from build123d import *

# Parameters (mm, degrees)
EXTRUDE_1_DEPTH = 3


with BuildPart() as part:
    # 草图1 → 凸台-拉伸1 (new body)
    with BuildSketch(Plane.XY):
        with BuildLine():
            Line((100.55, -11), (100.55, 11))
            Line((100.55, 11), (93.45, 11))
            ThreePointArc((93.45, 11), (92.4, 12.05), (93.45, 13.1))
            Line((93.45, 13.1), (93.45, 16))
            Line((93.45, 16), (49.05, 16))
            Line((49.05, 16), (49.05, 15.2))
            ThreePointArc((49.05, 15.2), (49.79246212, 14.89246212), (50.1, 14.15))
            ThreePointArc((50.1, 14.15), (49.79246212, 13.40753788), (49.05, 13.1))
            Line((49.05, 13.1), (45.95, 13.1))
            ThreePointArc((45.95, 13.1), (44.9, 14.15), (45.95, 15.2))
            Line((45.95, 15.2), (45.95, 16))
            Line((45.95, 16), (1.55, 16))
            Line((1.55, 16), (1.55, 13.1))
            ThreePointArc((1.55, 13.1), (2.29246212, 12.79246212), (2.6, 12.05))
            ThreePointArc((2.6, 12.05), (2.29246212, 11.30753788), (1.55, 11))
            Line((1.55, 11), (-5.55, 11))
            Line((-5.55, 11), (-5.55, -11))
            Line((-5.55, -11), (1.55, -11))
            ThreePointArc((1.55, -11), (2.29246212, -11.30753788), (2.6, -12.05))
            ThreePointArc((2.6, -12.05), (2.29246212, -12.79246212), (1.55, -13.1))
            Line((1.55, -13.1), (1.55, -16))
            Line((1.55, -16), (45.95, -16))
            Line((45.95, -16), (45.95, -15.2))
            ThreePointArc((45.95, -15.2), (44.9, -14.15), (45.95, -13.1))
            Line((45.95, -13.1), (49.05, -13.1))
            ThreePointArc((49.05, -13.1), (49.79246212, -13.40753788), (50.1, -14.15))
            ThreePointArc((50.1, -14.15), (49.79246212, -14.89246212), (49.05, -15.2))
            Line((49.05, -15.2), (49.05, -16))
            Line((49.05, -16), (93.45, -16))
            Line((93.45, -16), (93.45, -13.1))
            ThreePointArc((93.45, -13.1), (92.4, -12.05), (93.45, -11))
            Line((93.45, -11), (100.55, -11))
        make_face()
        with BuildLine():
            ThreePointArc((2.6, -4.05), (2.29246212, -4.79246212), (1.55, -5.1))
            Line((1.55, -5.1), (-1.55, -5.1))
            ThreePointArc((-1.55, -5.1), (-2.6, -4.05), (-1.55, -3))
            Line((-1.55, -3), (-1.55, 3))
            ThreePointArc((-1.55, 3), (-2.6, 4.05), (-1.55, 5.1))
            Line((-1.55, 5.1), (1.55, 5.1))
            ThreePointArc((1.55, 5.1), (2.29246212, 4.79246212), (2.6, 4.05))
            ThreePointArc((2.6, 4.05), (2.29246212, 3.30753788), (1.55, 3))
            Line((1.55, 3), (1.55, -3))
            ThreePointArc((1.55, -3), (2.29246212, -3.30753788), (2.6, -4.05))
        make_face(mode=Mode.SUBTRACT)
        Polygon((39.300498915, -12.5), (8.199501085, -12.5), (23.75, -1.819712284), align=None, mode=Mode.SUBTRACT)
        Polygon((55.699501085, -12.5), (71.25, -1.819712284), (86.800498915, -12.5), align=None, mode=Mode.SUBTRACT)
        with BuildLine():
            ThreePointArc((97.6, -4.05), (97.29246212, -4.79246212), (96.55, -5.1))
            Line((96.55, -5.1), (93.45, -5.1))
            ThreePointArc((93.45, -5.1), (92.4, -4.05), (93.45, -3))
            Line((93.45, -3), (93.45, 3))
            ThreePointArc((93.45, 3), (92.4, 4.05), (93.45, 5.1))
            Line((93.45, 5.1), (96.55, 5.1))
            ThreePointArc((96.55, 5.1), (97.29246212, 4.79246212), (97.6, 4.05))
            ThreePointArc((97.6, 4.05), (97.29246212, 3.30753788), (96.55, 3))
            Line((96.55, 3), (96.55, -3))
            ThreePointArc((96.55, -3), (97.29246212, -3.30753788), (97.6, -4.05))
        make_face(mode=Mode.SUBTRACT)
        Polygon((21.100498915, 0), (5.55, -10.680287716), (5.55, 10.680287716), align=None, mode=Mode.SUBTRACT)
        Polygon((26.399501085, 0), (41.95, 10.680287716), (41.95, -10.680287716), align=None, mode=Mode.SUBTRACT)
        Polygon((23.75, 1.819712284), (8.199501085, 12.5), (39.300498915, 12.5), align=None, mode=Mode.SUBTRACT)
        with BuildLine():
            ThreePointArc((50.1, -4.05), (49.79246212, -4.79246212), (49.05, -5.1))
            Line((49.05, -5.1), (45.95, -5.1))
            ThreePointArc((45.95, -5.1), (44.9, -4.05), (45.95, -3))
            Line((45.95, -3), (45.95, 3))
            ThreePointArc((45.95, 3), (44.9, 4.05), (45.95, 5.1))
            Line((45.95, 5.1), (49.05, 5.1))
            ThreePointArc((49.05, 5.1), (49.79246212, 4.79246212), (50.1, 4.05))
            ThreePointArc((50.1, 4.05), (49.79246212, 3.30753788), (49.05, 3))
            Line((49.05, 3), (49.05, -3))
            ThreePointArc((49.05, -3), (49.79246212, -3.30753788), (50.1, -4.05))
        make_face(mode=Mode.SUBTRACT)
        Polygon((53.05, 10.680287716), (68.600498915, 0), (53.05, -10.680287716), align=None, mode=Mode.SUBTRACT)
        Polygon((55.699501085, 12.5), (86.800498915, 12.5), (71.25, 1.819712284), align=None, mode=Mode.SUBTRACT)
        Polygon((89.45, 10.680287716), (89.45, -10.680287716), (73.899501085, 0), align=None, mode=Mode.SUBTRACT)
    extrude(amount=EXTRUDE_1_DEPTH)


solid = part.part
Input: part model. Units: mm. Frame: model coordinates. A direction names the side the tool comes from. Coordinates: 2 decimals unless noted, no trailing zeros. Order: outer loops, then holes, each group sorted by start corner. A loop starts at its lowest first (then second) coordinate and runs counter-clockwise, first axis right, second up. Notation, with made-up numbers: M -8.75,60 L 18.25,60 A36 ccw 18.25,94 Z; hole C 54.25,-32 d1. An arc over 180 degrees is marked long. Write item = value, one per line. Start each with the question number.
(1) Section C-C on z = 0.9. Give the number of separate pieces and of enclosed holes in the cut face, and give its area (3 significant figures).
(2) Reachability of faces 5 (the flat face through (-2, -11, 1)), 6 (the flat face through (48, 13.1, 1)), 7 (the flat face through (34.07, 5.27, 1.48)), 8 (the flat face through (23, -16, 1)) from +Z, -Z, +X, -X, +Y, -Y: full face, straight path, thin tool, end or side. Return the list, or none.
(3) Pull-direction query (Y, two-part tool) for faces 1 (the flat face through (97, 11, 1)), 2 (the flat face through (47, -13.1, 1)), 3 (the flat face through (45.95, 0, 1)), 4 (the flat face through (31.416, -7.085, 1.479)); classes: released by +Y, released by -Y, zero draft, split by the parting line, or undercut.
(4) Line query: line 1 along Y through (x, z) = (25.5, 0.4); line 2 along Y through (x, z) = (16, 0.6); line 3 along Y through (x, z) = (23, 0.55). Output: solid intervals per line, ascending. Write a range as [from, to].
(5) Section B-B on x = 73. Output: boundary loops of the cut face in (y, z), and give its area (3 significant figures).
(6) Section A-A on x = 36.5. Output: boundary loops of the cut face in (y, z).
(7) First-contact query: P1, Ø1.5, axis at y = 14, z = 2, coming from the +X side; P2, Ø1.5, axis at x = 98.5, z = 2, coming from the +Y side. Flat tips, straight axial feed; report the tip coordinate or a pass-through.
Result set:
q1.separate_pieces = 1
q1.enclosed_holes = 11
q1.area = 1,780 mm²
q2.face_5 = +Z, -Z, -X, -Y
q2.face_6 = +Z, -Z, +Y
q2.face_7 = +Z, -Z
q2.face_8 = +Z, -Z, +X, -X, -Y
q3.face_1 = released by +Y
q3.face_2 = released by -Y
q3.face_3 = undercut
q3.face_4 = undercut
q4.line_1 = [-16, -12.5], [-3.02, 3.02], [12.5, 16]
q4.line_2 = [-16, -12.5], [-7.14, -3.5], [3.5, 7.14], [12.5, 16]
q4.line_3 = [-16, -12.5], [-2.33, 2.33], [12.5, 16]
q5.outline = M -16,0 L -12.5,0 L -12.5,3 L -16,3 Z; M -3.02,0 L 3.02,0 L 3.02,3 L -3.02,3 Z; M 12.5,0 L 16,0 L 16,3 L 12.5,3 Z
q5.area = 39.1 mm²
q6.outline = M -16,0 L -12.5,0 L -12.5,3 L -16,3 Z; M -10.58,0 L -6.94,0 L -6.94,3 L -10.58,3 Z; M 6.94,0 L 10.58,0 L 10.58,3 L 6.94,3 Z; M 12.5,0 L 16,0 L 16,3 L 12.5,3 Z
q7.P1 = 93.45
q7.P2 = 11
